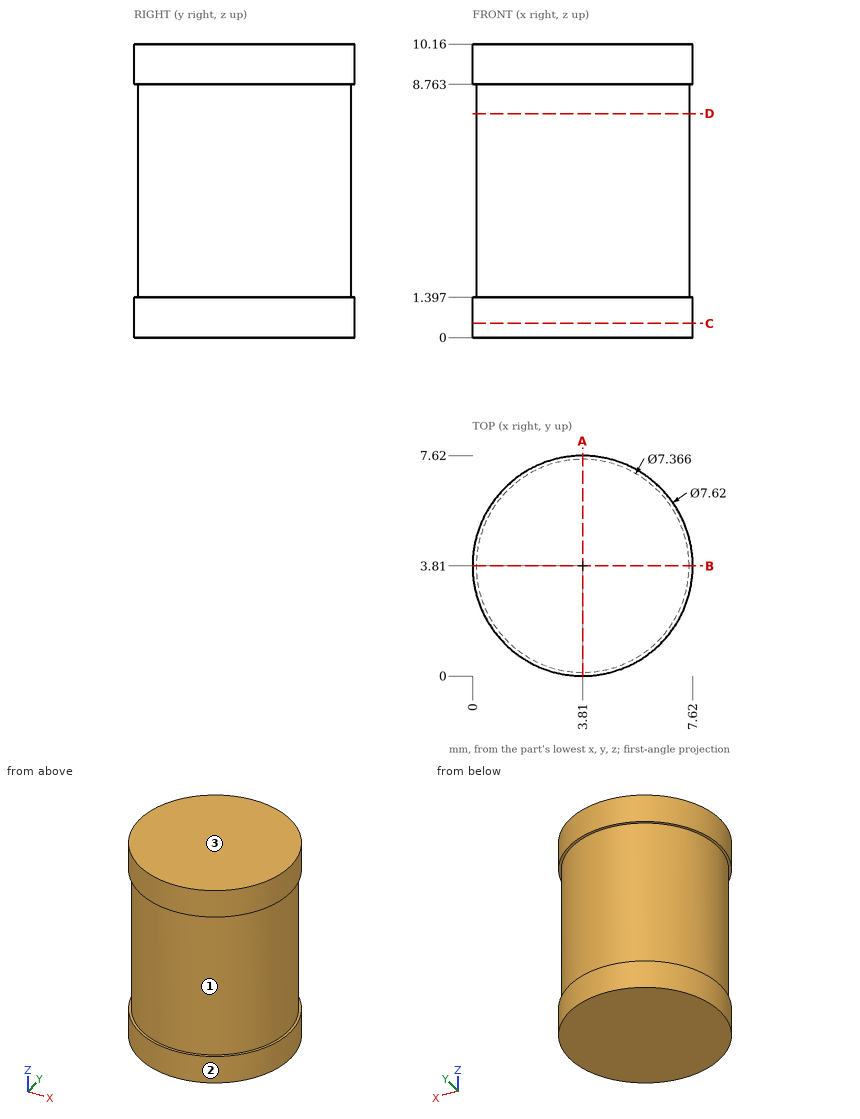
Geometry: see drawing. Coordinates: mm, zero at the bounding-box minimum. Give positions to 0.01 mm unless a question says otherwise; leave off trailing zeros. Write each loop counter-clockwise with the first axis right and the second up, starting at its lowest first coordinate (ties: lowest second). Pieces come first, ordered by that corner, then holes. Notation, with made-up numbers: M -39.75,50.5 L -4.75,50.5 A15 cw -4.75,65.5 Z; hole C 33.25,-16 d11. An arc over 180 degrees is marked long. Return JSON: item names as keys, results as strings. Group by question number.
1) Ray query, L1, parallel to Z at x = 1.25, y = 6.5; L2, parallel to X at y = 3.75, z = 1.75. Return the intervals inside material, ascending.
2) Cut plane C-C, the plane z = 0.5. Output: boundary loops of the cut face in (x, y).
3) Draft query along Z for the marked faces 1, 2 and 3. Return one class per face: released by +Z, released by -Z, zero draft, split by the parting line, or undercut.
4) Cut plane A-A, the plane x = 3.81. Output: boundary loops of the cut face in (y, z).
5) First-contact query: pin 1 Ø3 at (y, z) = (4.5, 6.5) entering from +X; pin 2 Ø1 at (y, z) = (1, 9) entering from -X; pin 3 Ø1 at (y, z) = (1.5, 1.5) entering from -X. Flat tips, straight axial feed; report the tip coordinate or a pass-through.
6) Cut plane D-D, the plane z = 7.75. Output: boundary loops of the cut face in (x, y), then the cut area to 3 significant figures.
Data:
{
 "1": {"L1": "z = 0 to 1.4, 8.76 to 10.16", "L2": "x = 0.13 to 7.49"},
 "2": {"outline": "C 3.81,3.81 d7.62"},
 "3": {"face 1": "undercut", "face 2": "zero draft", "face 3": "released by +Z"},
 "4": {"outline": "M 0,0 L 7.62,0 L 7.62,1.4 L 7.49,1.4 L 7.49,8.76 L 7.62,8.76 L 7.62,10.16 L 0,10.16 L 0,8.76 L 0.13,8.76 L 0.13,1.4 L 0,1.4 Z"},
 "5": {"pin 1": "stops at x = 7.49", "pin 2": "stops at x = 0.78", "pin 3": "stops at x = 0.46"},
 "6": {"outline": "C 3.81,3.81 d7.37", "area": "42.6 mm²"}
}
